For this review, use the dimensioned drawing (mm, ordinates from the lowest corner) and the shaded views. A direction names the side the tool comes from. Give positions to 0.01 mm unless a question says otherwise; leave off trailing zeros. Order: outer loops, then holes, each group sorted by start corner. A loop starts at its lowest first (then second) coordinate and runs counter-clockwise, first axis right, second up. Notation, with made-up numbers: (-31.5, -34.75) -> (22.5, -34.75) arc R16 cw to (22.5, -21.75) -> close; hole circle Ø2 at (8.25, 81). An arc over 180 degrees is marked (long way). Return JSON: item names as keys, results as strings.
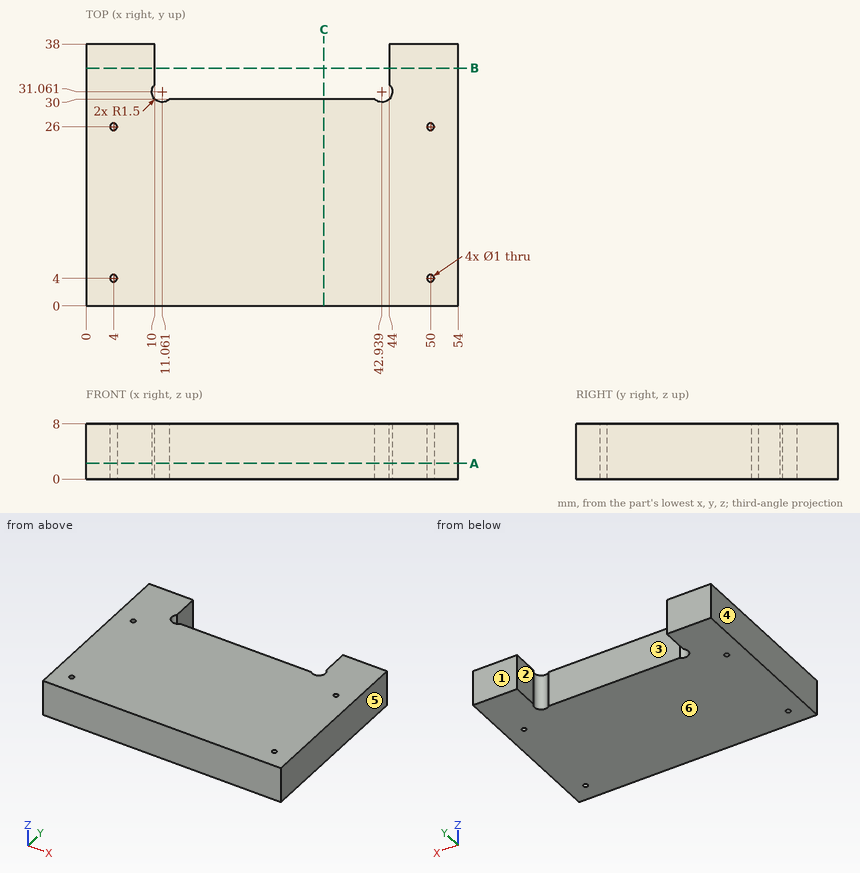
Item 1: Wall thickness on L1, parallel to X at y = 26, z = 6.25; L2, parallel to Y at x = 4, z = 5.25; L3, parallel to X at y = 34.5, z = 2.75: over which ranges is each line inside the solid? List them lowest first. Write a range as [from, to].
Result set:
{"L1": "x = [0, 3.5], [4.5, 49.5], [50.5, 54]", "L2": "y = [0, 3.5], [4.5, 25.5], [26.5, 38]", "L3": "x = [0, 10], [44, 54]"}
Item 2: Add section B-B (y = 34.5). Give the boundary of the cut face in (x, z), plus the area to 3 significant figures.
Result set:
{"outline": "(0, 0) -> (10, 0) -> (10, 8) -> (0, 8) -> close; (44, 0) -> (54, 0) -> (54, 8) -> (44, 8) -> close", "area": "160 mm^2"}
Item 3: Add section A-A (z = 2.25). Give the boundary of the cut face in (x, y), plus the area to 3 significant figures.
Result set:
{"outline": "(0, 0) -> (54, 0) -> (54, 38) -> (44, 38) -> (44, 32.12) arc R1.5 cw to (41.88, 30) -> (12.12, 30) arc R1.5 cw to (10, 32.12) -> (10, 38) -> (0, 38) -> close; hole circle Ø1 at (4, 4); hole circle Ø1 at (4, 26); hole circle Ø1 at (50, 4); hole circle Ø1 at (50, 26)", "area": "1,770 mm^2"}
Item 4: For pin 1 (4 mm diameter, centred on x = 29.5, z = 3.5, fed in from +Y), flat-tipped, find the tip position at first contact; note if it passes through.
Result set:
{"pin 1": "stops at y = 30"}
Item 5: Mouldability with a two-part tool opening along X and no side actions: class the marked faces 3, 4, 5 and 6 as released by +X, released by -X, zero draft, split by the parting line, or undercut.
Result set:
{"face 3": "undercut", "face 4": "released by -X", "face 5": "released by +X", "face 6": "zero draft"}
Item 6: Machinability: for the marked faces 1 and 2, which of the approach directions +Z, -Z, +X, -X, +Y, -Y give a long, thin tool a straight path to every point of the face, cutting with its end or side? Answer none if there is none.
Result set:
{"face 1": "+Z, -Z, +X, -X, +Y", "face 2": "+Z, -Z, +Y"}
Item 7: Add section C-C (x = 34.5). Give the boundary of the cut face in (y, z), plus the area to 3 significant figures.
Result set:
{"outline": "(0, 0) -> (30, 0) -> (30, 8) -> (0, 8) -> close", "area": "240 mm^2"}
